from build123d import *

# Parameters (mm, degrees)
F0_W     = 838.2
F0_H     = 304.8
F1_DEPTH = 19.05
F2_W     = 12.7
F2_H     = 12.7
F3_DEPTH = 838.201
F4_W     = 12.7
F4_H     = 6.35
F5_DEPTH = 304.801


with BuildPart() as f1:
    # F0 (on Front) → F1 (new body)
    with BuildSketch(Plane.XZ):
        with Locations((419.1, 152.4)):
            Rectangle(F0_W, F0_H)
    extrude(amount=F1_DEPTH)

    # F2 (on face) → F3 (cut, through all)
    with BuildSketch(Plane.YZ.offset(838.2)):
        with Locations((-12.7, 6.35)):
            Rectangle(F2_W, F2_H)
    extrude(amount=-F3_DEPTH, mode=Mode.SUBTRACT)

    # F4 (on face) → F5 (cut, through all)
    with BuildSketch(Plane.XY.offset(304.8)):
        with Locations((831.85, -15.875)):
            Rectangle(F4_W, F4_H)
        with Locations((6.35, -15.875)):
            Rectangle(F4_W, F4_H)
    extrude(amount=-F5_DEPTH, mode=Mode.SUBTRACT)


solid = f1.part
Could you check a few things on this model? Use its own coordinates, in mm. Round coordinates to 2 decimals unless told otherwise and drop trailing zeros. Write each loop counter-clockwise with the first axis right and the second up, starting at its lowest first coordinate (ties: lowest second). Pieces come first, ordered by that corner, then holes. Notation, with made-up numbers: (42, 24.5) - (62, 24.5) arc R20 ccw to (62, 58.5) - close; hole circle Ø10 at (-10, -2.75). An arc over 180 degrees is marked (long way). Use a Markdown table: item, result.
Q1. I want a section at B-B (y = -16). List the corners of the cut face in (x, z) for me, plus the area to 3 significant figures.
Output values:
| item | result |
|---|---|
| outline | (12.7, 12.7) - (825.5, 12.7) - (825.5, 304.8) - (12.7, 304.8) - close |
| area | 237,000 mm2 |
Q2. I want a section at A-A (x = 777). List the corners of the cut face in (y, z) for me.
Output values:
| item | result |
|---|---|
| outline | (-19.05, 12.7) - (-6.35, 12.7) - (-6.35, 0) - (0, 0) - (0, 304.8) - (-19.05, 304.8) - close |
Q3. Please list where these lines run through material, in increasing order: L1, parallel to Z at x = 232, y = -12; L2, parallel to X at y = -14.75, z = 149.5.
Output values:
| item | result |
|---|---|
| L1 | 12.7 to 304.8 |
| L2 | 12.7 to 825.5 |
Q4. For pin 1 (10 mm diameter, centred on x = 5, z = 101.5, fed in from -Y); pin 2 (1 mm diameter, centred on x = 140.5, y = -15.5, fed in from -Z); pin 3 (7 mm diameter, centred on y = -15, z = 228.5, fed in from +X); pin 4 (4 mm diameter, centred on x = 286.5, z = 6.5, fed in from -Y), each with a flat end and sliding along its axis, tell me the tip position at first contact or that it passes through.
Output values:
| item | result |
|---|---|
| pin 1 | y = -12.7 |
| pin 2 | z = 12.7 |
| pin 3 | x = 838.2 |
| pin 4 | y = -6.35 |
